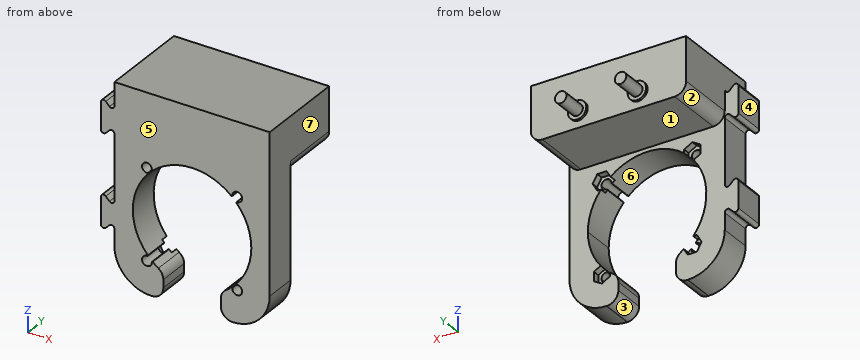
```python
from build123d import *

# Parameters (mm, degrees)
SKETCH1_W           = 67.5
SKETCH1_H           = 85.123863618
BOSS_EXTRUDE1_DEPTH = 14
SKETCH2_W           = 67.5
SKETCH2_H           = 24
BOSS_EXTRUDE2_DEPTH = 26
SKETCH3_R           = 2.5
BOSS_EXTRUDE3_DEPTH = 12
FILLET1_R           = 0.25
SKETCH4_R           = 4
BOSS_EXTRUDE4_DEPTH = 1
SKETCH5_W           = 25
SKETCH5_H           = 20
CUT_EXTRUDE1_DEPTH  = 81.512957839
FILLET2_R           = 5
FILLET3_R           = 16
BOSS_EXTRUDE5_DEPTH = 14
CUT_EXTRUDE2_DEPTH  = 84.206588569
FILLET4_START       = -1
FILLET4_DEPTH       = 15
FILLET4_2_DEPTH     = 14
CUT_EXTRUDE3_DEPTH  = 3
CIRPATTERN1_COUNT   = 4


with BuildPart() as part:
    # Sketch1 → Boss-Extrude1 (new body)
    with BuildSketch(Plane(origin=(0, 0, 0), x_dir=(1, 0, 0), z_dir=(0, 1, 0))):
        with Locations((0, -8.811931809)):
            Rectangle(SKETCH1_W, SKETCH1_H)
        with BuildLine():
            ThreePointArc((18.737427526, 17.66270958), (23.93273134, 9.50194036), (25.75, 0))
            ThreePointArc((25.75, 0), (23.93273134, -9.50194036), (18.737427526, -17.66270958))
            ThreePointArc((18.737427526, -17.66270958), (20.788448756, -17.816003175), (21.772213178, -19.622213178))
            ThreePointArc((21.772213178, -19.622213178), (19.169682922, -21.724049605), (17.66270958, -18.737427526))
            ThreePointArc((17.66270958, -18.737427526), (0, -25.75), (-17.66270958, -18.737427526))
            ThreePointArc((-17.66270958, -18.737427526), (-17.52037675, -19.169682922), (-17.472213178, -19.622213178))
            ThreePointArc((-17.472213178, -19.622213178), (-21.428423181, -20.788448756), (-18.737427526, -17.66270958))
            ThreePointArc((-18.737427526, -17.66270958), (-25.75, 0), (-18.737427526, 17.66270958))
            ThreePointArc((-18.737427526, 17.66270958), (-21.428423181, 20.788448756), (-17.472213178, 19.622213178))
            ThreePointArc((-17.472213178, 19.622213178), (-17.52037675, 19.169682922), (-17.66270958, 18.737427526))
            ThreePointArc((-17.66270958, 18.737427526), (0, 25.75), (17.66270958, 18.737427526))
            ThreePointArc((17.66270958, 18.737427526), (19.169682922, 21.724049605), (21.772213178, 19.622213178))
            ThreePointArc((21.772213178, 19.622213178), (20.788448756, 17.816003175), (18.737427526, 17.66270958))
        make_face(mode=Mode.SUBTRACT)
    extrude(amount=BOSS_EXTRUDE1_DEPTH)

    # Sketch2 → Boss-Extrude2 (add)
    with BuildSketch(Plane(origin=(0, 14, 0), x_dir=(1, 0, 0), z_dir=(0, 1, 0))):
        with Locations((0, -39.373863618)):
            Rectangle(SKETCH2_W, SKETCH2_H)
    extrude(amount=BOSS_EXTRUDE2_DEPTH)

    # Sketch3 → Boss-Extrude3 (add)
    with BuildSketch(Plane(origin=(0, 40, 0), x_dir=(1, 0, 0), z_dir=(0, 1, 0))):
        with Locations(Location((13, -34.373863618, 0), (0, 0, 270))):
            Circle(SKETCH3_R)
        with Locations(Location((-13, -34.373863618, 0), (0, 0, 270))):
            Circle(SKETCH3_R)
    extrude(amount=BOSS_EXTRUDE3_DEPTH)

    # Fillet1
    fillet1_edges = [part.edges().sort_by_distance(p)[0] for p in [
        (-17.66270958, 7, 18.737427526),
        (17.66270958, 7, 18.737427526),
        (18.737427526, 7, 17.66270958),
        (18.737427526, 7, -17.66270958),
        (17.66270958, 7, -18.737427526),
        (-17.66270958, 7, -18.737427526),
        (-18.737427526, 7, -17.66270958),
        (-18.737427526, 7, 17.66270958),
    ]]
    fillet(fillet1_edges, radius=FILLET1_R)

    # Sketch4 → Boss-Extrude4 (add)
    with BuildSketch(Plane(origin=(0, 40, 0), x_dir=(1, 0, 0), z_dir=(0, 1, 0))):
        with Locations(Location((13, -34.373863618, 0), (0, 0, 270))):
            Circle(SKETCH4_R)
        with Locations(Location((-13, -34.373863618, 0), (0, 0, 270))):
            Circle(SKETCH4_R)
    extrude(amount=BOSS_EXTRUDE4_DEPTH)

    # Sketch5 → Cut-Extrude1 (cut, through all)
    with BuildSketch(Plane.XZ):
        with Locations((0, -23.75)):
            Rectangle(SKETCH5_W, SKETCH5_H)
    extrude(amount=-CUT_EXTRUDE1_DEPTH, mode=Mode.SUBTRACT)

    # Fillet2
    fillet2_edges = [part.edges().sort_by_distance(p)[0] for p in [
        (12.5, 7, -22.51249653),
        (-12.5, 7, -22.51249653),
        (12.5, 7, -33.75),
        (-12.5, 7, -33.75),
        (-33.75, 27, 27.373863618),
        (33.75, 27, 27.373863618),
    ]]
    fillet(fillet2_edges, radius=FILLET2_R)

    # Fillet3
    fillet3_edges = [part.edges().sort_by_distance(p)[0] for p in [
        (33.75, 7, -33.75),
        (-33.75, 7, -33.75),
    ]]
    fillet(fillet3_edges, radius=FILLET3_R)

    # Sketch6 → Boss-Extrude5 (add)
    with BuildSketch(Plane.XZ):
        Polygon((-33.75, 38.373863618), (-39.75, 44.373863618), (-39.75, 26.373863618), (-33.75, 32.373863618), align=None)
        Polygon((-39.75, 4.373863618), (-33.75, -1.626136382), (-33.75, -7.626136382), (-39.75, -13.626136382), align=None)
    extrude(amount=-BOSS_EXTRUDE5_DEPTH)

    # Sketch7 → Cut-Extrude2 (cut, through all)
    with BuildSketch(Plane.XZ):
        Polygon((-33.75, -7.626136382), (-33.75, -7.512999297), (-39.67, -13.432999297), (-39.67, 4.180726533), (-33.75, -1.739273467), (-33.75, -1.626136382), (-39.75, 4.373863618), (-39.75, -13.626136382), align=None)
        Polygon((-33.75, 32.373863618), (-33.75, 32.487000703), (-39.67, 26.567000703), (-39.67, 44.180726533), (-33.75, 38.260726533), (-33.75, 38.373863618), (-39.75, 44.373863618), (-39.75, 26.373863618), align=None)
    extrude(amount=-CUT_EXTRUDE2_DEPTH, mode=Mode.SUBTRACT)

    # Fillet4: read off the stored shape, not the designer's step
    # Fillet4 outline → Fillet4 (cut)
    with BuildSketch(Plane(origin=(0, 0, 0), x_dir=(1, 0, 0), z_dir=(0, 1, 0)).offset(FILLET4_START)):
        with BuildLine():
            Line((-39.67, -26.567000703), (-39.67, -29.584767656))
            ThreePointArc((-39.67, -29.584767656), (-38.898354291, -28.42991824), (-37.536116524, -28.700884179))
            Line((-37.536116524, -28.700884179), (-39.67, -26.567000703))
        make_face()
        with BuildLine():
            Line((-39.67, 13.432999297), (-39.67, 10.415232344))
            ThreePointArc((-39.67, 10.415232344), (-38.898354291, 11.57008176), (-37.536116524, 11.299115821))
            Line((-37.536116524, 11.299115821), (-39.67, 13.432999297))
        make_face()
        with BuildLine():
            Line((-39.67, -4.180726533), (-37.536116524, -2.046843056))
            ThreePointArc((-37.536116524, -2.046843056), (-38.89835429, -2.317808995), (-39.67, -1.16295958))
            Line((-39.67, -1.16295958), (-39.67, -4.180726533))
        make_face()
        with BuildLine():
            ThreePointArc((-37.536116524, -42.046843056), (-38.89835429, -42.317808995), (-39.67, -41.16295958))
            Line((-39.67, -41.16295958), (-39.67, -44.180726533))
            Line((-39.67, -44.180726533), (-37.536116524, -42.046843056))
        make_face()
    extrude(amount=FILLET4_DEPTH, mode=Mode.SUBTRACT)

    # Fillet4 2 outline → Fillet4 2 (add)
    with BuildSketch(Plane(origin=(0, 0, 0), x_dir=(1, 0, 0), z_dir=(0, 1, 0))):
        with BuildLine():
            ThreePointArc((-33.75, 10.53076625), (-34.52164571, 9.375916835), (-35.883883476, 9.646882774))
            Line((-35.883883476, 9.646882774), (-33.75, 7.512999297))
            Line((-33.75, 7.512999297), (-33.75, 10.53076625))
        make_face()
        with BuildLine():
            ThreePointArc((-35.883883476, -0.394610009), (-34.521645709, -0.12364407), (-33.75, -1.278493486))
            Line((-33.75, -1.278493486), (-33.75, 1.739273467))
            Line((-33.75, 1.739273467), (-35.883883476, -0.394610009))
        make_face()
        with BuildLine():
            ThreePointArc((-33.75, -29.46923375), (-34.52164571, -30.624083165), (-35.883883476, -30.353117226))
            Line((-35.883883476, -30.353117226), (-33.75, -32.487000703))
            Line((-33.75, -32.487000703), (-33.75, -29.46923375))
        make_face()
        with BuildLine():
            Line((-33.75, -38.260726533), (-35.883883476, -40.394610009))
            ThreePointArc((-35.883883476, -40.394610009), (-34.521645709, -40.12364407), (-33.75, -41.278493486))
            Line((-33.75, -41.278493486), (-33.75, -38.260726533))
        make_face()
    extrude(amount=FILLET4_2_DEPTH)

    # Sketch8 → Cut-Extrude3 (cut)
    with BuildSketch(Plane(origin=(0, 14, 0), x_dir=(1, 0, 0), z_dir=(0, 1, 0))):
        Polygon((-19.622213178, -15.580761294), (-16.122213178, -17.601487236), (-16.122213178, -21.64293912), (-19.622213178, -23.663665062), (-23.122213178, -21.64293912), (-23.122213178, -17.601487236), align=None)
    cut_extrude3 = extrude(amount=-CUT_EXTRUDE3_DEPTH, mode=Mode.SUBTRACT)

    # CirPattern1: Cut-Extrude3 ×4 about axis
    cirpattern1_axis = Axis((0, 0, 0), (0, 1, 0))
    for i in range(1, CIRPATTERN1_COUNT):
        add(cut_extrude3.rotate(cirpattern1_axis, i * 360 / CIRPATTERN1_COUNT), mode=Mode.SUBTRACT)


solid = part.part
```
Build history of the part. All positions in model axes, mm. Face numbers are marked on the shaded views. A direction names the side the tool comes from. Give positions to 0.01 mm unless a question says otherwise; leave off trailing zeros. Loops run counter-clockwise (first coordinate to the right, second up) from the corner with the lowest first, then second, coordinate; pieces in that order, holes last. Notation, with made-up numbers: (-22, 29.5) - (34, 29.5) arc R14 cw to (34, 35.5) - close; hole circle Ø3 at (75.5, -27). An arc over 180 degrees is marked (long way). Use a Markdown table: item, result.
(1) Band-saw the part on B-B (z = 6). Give the cut face in (x, y).
Taken from the geometry:
| item | result |
|---|---|
| outline | (-33.75, 0) - (-25.04, 0) - (-25.04, 14) - (-33.75, 14) - close; (25.04, 0) - (33.75, 0) - (33.75, 14) - (25.04, 14) - close |
(2) Band-saw the part on A-A (y = 43). Give the cut face in (x, z), and give its area (3 significant figures).
Taken from the geometry:
| item | result |
|---|---|
| outline | circle Ø5 at (-13, 34.37); circle Ø5 at (13, 34.37) |
| area | 39.3 mm2 |
(3) Wall check: line 1 along Z through (x, y) = (-10.5, 16.5); line 2 along Y through (x, z) = (-23, -30); line 3 along X through (y, z) = (9, 1.5). Give the ranges that are in metal, low to high.
Taken from the geometry:
| item | result |
|---|---|
| line 1 | 27.37 to 51.37 |
| line 2 | 0 to 14 |
| line 3 | -39.62 to -36.99, -33.75 to -25.71, 25.71 to 33.75 |
(4) Drop flat-ended pins along their axis: pin 1 Ø2.5 at (x, y) = (20, 13) entering from -Z; pin 2 Ø1.7 at (y, z) = (7, -27) entering from +X; pin 3 Ø1 at (y, z) = (8, -27) entering from -X. Give the stop position or say it passes through.
Taken from the geometry:
| item | result |
|---|---|
| pin 1 | z = -33.72 |
| pin 2 | x = 31.37 |
| pin 3 | x = -31.15 |
(5) Which spindle directions (+Z, -Z, +X, -X, +Y, -Y) get a long thin tool onto all of the face, cutting with end or side? Do the marked faces 1, 2 and 3. Say none if no direction does.
Taken from the geometry:
| item | result |
|---|---|
| face 1 | -Z, +X, -X, +Y |
| face 2 | -Z, -X, +Y |
| face 3 | -Z, +Y, -Y |
(6) Pull direction X, two halves, no side cores. Call the marked faces 4, 5, 6 and 7: +X half, -X half, draft (parallel to the pull), parting line (faces both ways), or undercut.
Taken from the geometry:
| item | result |
|---|---|
| face 4 | -X half |
| face 5 | draft |
| face 6 | undercut |
| face 7 | +X half |
(7) Band-saw the part on C-C (y = 27.5). Give the cut face in (x, z), and give its area (3 significant figures).
Taken from the geometry:
| item | result |
|---|---|
| outline | (-33.75, 32.37) arc R5 ccw to (-28.75, 27.37) - (28.75, 27.37) arc R5 ccw to (33.75, 32.37) - (33.75, 51.37) - (-33.75, 51.37) - close |
| area | 1,610 mm2 |
(8) Band-saw the part on D-D (z = 44). Give the cut face in (x, y).
Taken from the geometry:
| item | result |
|---|---|
| outline | (-33.75, 0) - (33.75, 0) - (33.75, 40) - (-33.75, 40) - close |
